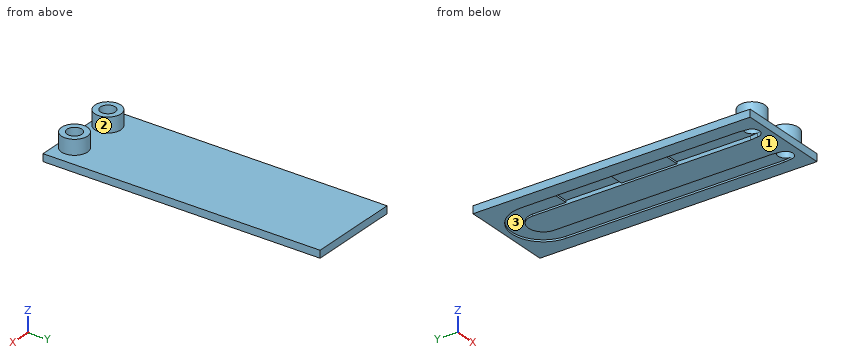
```python
from build123d import *

# Parameters (mm, degrees)
F0_W      = 25
F0_H      = 75
F3_DEPTH  = 2
F4_DEPTH  = 0.5
F6_R      = 3.5
F6_R_2    = 2
F7_DEPTH  = 4
F8_DEPTH  = 1
F9_W      = 4.5
F9_H      = 15
F10_DEPTH = 1
F11_DEPTH = 2


with BuildPart() as f3:
    # F0 (on Top) → F3 (new body)
    with BuildSketch(Plane.XY):
        with Locations((-31.788486, -12.391831)):
            Rectangle(F0_W, F0_H)
    extrude(amount=F3_DEPTH)

    # F1 (on face) → F4 (cut)
    with BuildSketch(Plane.XY):
        with BuildLine():
            ThreePointArc((-27.538486, -45.891831), (-25.538486, -47.891831), (-23.538486, -45.891831))
            ThreePointArc((-23.538486, -45.891831), (-25.538486, -43.891831), (-27.538486, -45.891831))
        make_face()
        with BuildLine():
            ThreePointArc((-27.538486, -45.891831), (-25.538486, -43.891831), (-23.538486, -45.891831))
            Line((-23.538486, -45.891831), (-23.288486, -43.891831))
            Line((-23.288486, -43.891831), (-23.288486, 15.108169))
            ThreePointArc((-23.288486, 15.108169), (-31.788486, 23.608169), (-40.288486, 15.108169))
            Line((-40.288486, 15.108169), (-40.288486, -43.891831))
            Line((-40.288486, -43.891831), (-40.038486, -45.891831))
            ThreePointArc((-40.038486, -45.891831), (-38.038486, -43.891831), (-36.038486, -45.891831))
            Line((-36.038486, -45.891831), (-35.788486, -43.891831))
            Line((-35.788486, -43.891831), (-35.788486, 15.108169))
            ThreePointArc((-35.788486, 15.108169), (-31.788486, 19.108169), (-27.788486, 15.108169))
            Line((-27.788486, 15.108169), (-27.788486, -43.891831))
            Line((-27.788486, -43.891831), (-27.538486, -45.891831))
        make_face()
        with BuildLine():
            ThreePointArc((-36.038486, -45.891831), (-38.038486, -43.891831), (-40.038486, -45.891831))
            ThreePointArc((-40.038486, -45.891831), (-38.038486, -47.891831), (-36.038486, -45.891831))
        make_face()
    extrude(amount=F4_DEPTH, mode=Mode.SUBTRACT)

    # F6 (on face) → F7 (join)
    with BuildSketch(Plane.XY.offset(2)):
        with Locations((-38.038486, -45.891831)):
            Circle(F6_R)
        with Locations((-38.038486, -45.891831)):
            Circle(F6_R_2, mode=Mode.SUBTRACT)
        with Locations((-25.538486, -45.891831)):
            Circle(F6_R)
        with Locations((-25.538486, -45.891831)):
            Circle(F6_R_2, mode=Mode.SUBTRACT)
    extrude(amount=F7_DEPTH)

    # F6 (on face) → F8 (cut)
    with BuildSketch(Plane.XY.offset(2)):
        with Locations((-25.538486, -45.891831)):
            Circle(F6_R_2)
        with Locations((-38.038486, -45.891831)):
            Circle(F6_R_2)
    extrude(amount=-F8_DEPTH, mode=Mode.SUBTRACT)

    # F9 (on face) → F10 (cut)
    with BuildSketch(Plane.XY):
        with BuildLine():
            Line((-40.288486, -43.891831), (-40.038486, -45.891831))
            ThreePointArc((-40.038486, -45.891831), (-38.038486, -47.891831), (-36.038486, -45.891831))
            Line((-36.038486, -45.891831), (-35.788486, -43.891831))
            Line((-35.788486, -43.891831), (-35.788486, -23.891831))
            Line((-35.788486, -23.891831), (-40.288486, -23.891831))
            Line((-40.288486, -23.891831), (-40.288486, -43.891831))
        make_face()
        with Locations((-38.038486, -1.391831)):
            Rectangle(F9_W, F9_H)
    extrude(amount=F10_DEPTH, mode=Mode.SUBTRACT)

    # F6 (on face) → F11 (cut)
    with BuildSketch(Plane.XY.offset(2)):
        with Locations((-25.538486, -45.891831)):
            Circle(F6_R_2)
        with Locations((-38.038486, -45.891831)):
            Circle(F6_R_2)
    extrude(amount=-F11_DEPTH, mode=Mode.SUBTRACT)


solid = f3.part
```
Read the model definition and answer for the solid it produces. Units are mm, in the model's axes. Face numbers are marked on the shaded views. Round coordinates to 2 decimals unless told otherwise and drop trailing zeros. Write each loop counter-clockwise with the first axis right and the second up, starting at its lowest first coordinate (ties: lowest second). Pieces come first, ordered by that corner, then holes. Notation, with made-up numbers: (41, 77.25) -> (89, 77.25) arc R35 ccw to (89, 113.25) -> close; hole circle Ø5 at (3.25, 64.5). An arc over 180 degrees is marked (long way). Answer in a Markdown table with one row per item. Add a question column.
1) Find section C-C, the plane x = -37.75. Determine the outline of the cut face in (y, z).
2) Find section B-B, the plane z = 3.35. Determine the outline of the cut face in (x, y).
3) Find section A-A, the plane y = 0.5. Determine the outline of the cut face in (x, z).
4) Given P1, Ø12, axis at x = -38.5, y = -39.5, coming from the +Z side; P2, Ø1.3, axis at x = -39, y = -0.5, coming from the -Z side; P3, Ø7.5, axis at x = -38, y = -28, coming from the +Z side; P4, Ø1.3, axis at x = -39, y = -14, coming from the -Z side, each flat-ended and moving along its own axis, determine where each tip first touches the part or whether it passes through.
5) Determine the mould class of the marked faces 1, 2 and 3 for opening direction Y: pulls with the +Y half, pulls with the -Y half, needs draft (parallel to the pull), parting line crosses it, or undercut.
6) Consider line 1 (Y direction, x = -38, z = 2.8); line 2 (X direction, y = 6.5, z = 0.35); line 3 (Z direction, x = -28.5, y = 8.5). Determine where each line is inside the solid, lowest interval first.
7) Find section D-D, the plane x = -26.25. Determine the outline of the cut face in (y, z).
Findings below:
| question | item | result |
|---|---|---|
| 1 | outline | (-49.89, 0) -> (-47.87, 0) -> (-47.87, 6) -> (-49.38, 6) -> (-49.38, 2) -> (-49.89, 2) -> close; (-43.91, 1) -> (-23.89, 1) -> (-23.89, 0.5) -> (-8.89, 0.5) -> (-8.89, 1) -> (6.11, 1) -> (6.11, 0.5) -> (21.17, 0.5) -> (21.17, 0) -> (25.11, 0) -> (25.11, 2) -> (-42.4, 2) -> (-42.4, 6) -> (-43.91, 6) -> close |
| 2 | outline | circle Ø7 at (-38.04, -45.89); circle Ø7 at (-25.54, -45.89); hole circle Ø4 at (-38.04, -45.89); hole circle Ø4 at (-25.54, -45.89) |
| 3 | outline | (-44.29, 0) -> (-40.29, 0) -> (-40.29, 1) -> (-35.79, 1) -> (-35.79, 0) -> (-27.79, 0) -> (-27.79, 0.5) -> (-23.29, 0.5) -> (-23.29, 0) -> (-19.29, 0) -> (-19.29, 2) -> (-44.29, 2) -> close |
| 4 | P1 | z = 6 |
| 4 | P2 | z = 1 |
| 4 | P3 | z = 2 |
| 4 | P4 | z = 0.5 |
| 5 | face 1 | needs draft |
| 5 | face 2 | parting line crosses it |
| 5 | face 3 | undercut |
| 6 | line 1 | -49.39 to -47.89, -43.89 to -42.39 |
| 6 | line 2 | -44.29 to -40.29, -35.79 to -27.79, -23.29 to -19.29 |
| 6 | line 3 | 0 to 2 |
| 7 | outline | (-49.89, 0) -> (-47.76, 0) -> (-47.76, 6) -> (-49.32, 6) -> (-49.32, 2) -> (-49.89, 2) -> close; (-44.02, 0.5) -> (21.56, 0.5) -> (21.56, 0) -> (25.11, 0) -> (25.11, 2) -> (-42.46, 2) -> (-42.46, 6) -> (-44.02, 6) -> close |
